```python
from build123d import *

# Parameters (mm, degrees)
SKETCH1_R           = 60
BOSS_EXTRUDE1_DEPTH = 60
SKETCH2_R           = 30
CUT_EXTRUDE1_DEPTH  = 40
SKETCH3_R           = 10
CUT_EXTRUDE2_DEPTH  = 40
SKETCH4_R           = 5
CUT_EXTRUDE3_DEPTH  = 100
SKETCH5_R           = 5
CUT_EXTRUDE4_DEPTH  = 100
CUT_EXTRUDE5_DEPTH  = 20


with BuildPart() as part:
    # Sketch1 → Boss-Extrude1 (new body)
    with BuildSketch(Plane.XY):
        Circle(SKETCH1_R)
    extrude(amount=BOSS_EXTRUDE1_DEPTH)

    # Sketch2 → Cut-Extrude1 (cut)
    with BuildSketch(Plane.XY.offset(60)):
        Circle(SKETCH2_R)
    extrude(amount=-CUT_EXTRUDE1_DEPTH, mode=Mode.SUBTRACT)

    # Sketch3 → Cut-Extrude2 (cut)
    with BuildSketch(Plane.XY.offset(20)):
        Circle(SKETCH3_R)
    extrude(amount=-CUT_EXTRUDE2_DEPTH, mode=Mode.SUBTRACT)

    # Sketch4 → Cut-Extrude3 (cut)
    with BuildSketch(Plane.XY.offset(60)):
        with Locations((0, 45)):
            Circle(SKETCH4_R)
    extrude(amount=-CUT_EXTRUDE3_DEPTH, mode=Mode.SUBTRACT)

    # Sketch5 → Cut-Extrude4 (cut)
    with BuildSketch(Plane.XY.offset(60)):
        with Locations((-40, -20)):
            Circle(SKETCH5_R)
        with Locations((40, -20)):
            Circle(SKETCH5_R)
    extrude(amount=-CUT_EXTRUDE4_DEPTH, mode=Mode.SUBTRACT)

    # Sketch6 → Cut-Extrude5 (cut)
    with BuildSketch(Plane.XY.offset(60)):
        with BuildLine():
            Line((-20, 56.568542495), (-20, 22.360679775))
            ThreePointArc((-20, 22.360679775), (0.705121947, 29.991712239), (21.02874571, 21.396070991))
            Line((21.02874571, 21.396070991), (21.02874571, 56.194233279))
            ThreePointArc((21.02874571, 56.194233279), (0.547363025, 59.997503229), (-20, 56.568542495))
        make_face()
    extrude(amount=-CUT_EXTRUDE5_DEPTH, mode=Mode.SUBTRACT)


solid = part.part
```
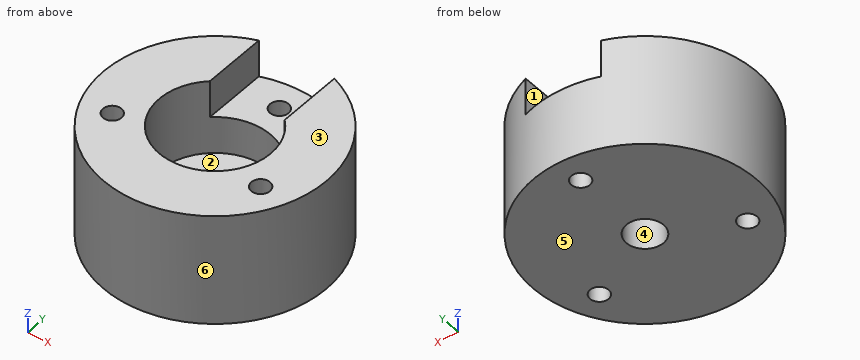
Geometry check sheet. Reference: the model listing, model coordinates, mm. Face numbers are marked on the shaded views. A direction names the side the tool comes from. Give positions to 0.01 mm unless a question says otherwise; leave off trailing zeros. Order: outer loops, then holes, each group sorted by start corner. A loop starts at its lowest first (then second) coordinate and runs counter-clockwise, first axis right, second up.
1. Section check D-D, the plane z = 54. Enter the section's corners in (x, y).
2. Release check for a two-part mould opening along Y. For the marked faces 4, 5 and 6 record: pulls with the +Y half, pulls with the -Y half, needs draft (parallel to the pull), parting line crosses it, or undercut.
3. Section check B-B, the plane x = 0. Enter the section's corners in (y, z), and give its area (3 significant figures).
4. Section check A-A, the plane y = 0. Enter the section's corners in (x, z).
5. Thickness scan on L1, parallel to Y at x = 0, z = 5; L2, parallel to X at y = -1, z = 34.5; L3, parallel to Z at x = 5.5, y = 15.5. Record the ranges inside material, lowest first.
6. Access from +Z, -Z, +X, -X, +Y, -Y to the whole of each face (thin tool, end or side, straight path). Record for the marked faces 1, 2 and 3.
7. Gauge pin test, flat ends, axial feed: pin 1 Ø8 at (x, z) = (15.5, 51) entering from +Y; pin 2 Ø18 at (x, y) = (-7, -13) entering from +Z; pin 3 Ø4 at (x, z) = (3, 35) entering from -Y. Record the tip position at first contact, or that the pin passes through.
8. Section check C-C, the plane y = -20. Enter the section's corners in (x, z), and give its area (3 significant figures).
Values follow:
1. outline: (-20, 22.36) - (-20, 56.57) arc R60 ccw (long way) to (21.03, 56.19) - (21.03, 21.4) arc R30 cw (long way) to start; hole circle Ø10 at (-40, -20); hole circle Ø10 at (40, -20)
2. face 4: undercut
2. face 5: needs draft
2. face 6: parting line crosses it
3. outline: (-60, 0) - (-10, 0) - (-10, 20) - (-30, 20) - (-30, 60) - (-60, 60) - close; (10, 0) - (40, 0) - (40, 40) - (30, 40) - (30, 20) - (10, 20) - close; (50, 0) - (60, 0) - (60, 40) - (50, 40) - close
3. area: 3,400 mm2
4. outline: (-60, 0) - (-10, 0) - (-10, 20) - (-30, 20) - (-30, 60) - (-60, 60) - close; (10, 0) - (60, 0) - (60, 60) - (30, 60) - (30, 20) - (10, 20) - close
5. L1: y = -60 to -10, 10 to 40, 50 to 60
5. L2: x = -59.99 to -29.98, 29.98 to 59.99
5. L3: z = 0 to 20
6. face 1: +Z, +Y
6. face 2: +Z
6. face 3: +Z, +X, -X, +Y, -Y
7. pin 1: stops at y = -22.8
7. pin 2: stops at z = 20
7. pin 3: stops at y = -59.99
8. outline: (-56.57, 0) - (-45, 0) - (-45, 60) - (-56.57, 60) - close; (-35, 0) - (35, 0) - (35, 60) - (22.36, 60) - (22.36, 20) - (-22.36, 20) - (-22.36, 60) - (-35, 60) - close; (45, 0) - (56.57, 0) - (56.57, 60) - (45, 60) - close
8. area: 3,800 mm2
